```python
from build123d import *

# Parameters (mm, degrees)
SKETCH1_R           = 4.75
BOSS_EXTRUDE1_DEPTH = 5
SKETCH2_R           = 2.25
BOSS_EXTRUDE2_DEPTH = 7.5
BOSS_EXTRUDE3_START = 12.5
SKETCH3_R           = 2.25
BOSS_EXTRUDE3_DEPTH = 12.5
SKETCH4_R           = 1.25
CUT_EXTRUDE1_DEPTH  = 5
CUT_EXTRUDE2_START  = -5
SKETCH5_R           = 1.25
CUT_EXTRUDE2_DEPTH  = 5


with BuildPart() as part:
    # Sketch1 → Boss-Extrude1 (new body)
    with BuildSketch(Plane.XY):
        Circle(SKETCH1_R)
    extrude(amount=BOSS_EXTRUDE1_DEPTH)

    # Sketch2 → Boss-Extrude2 (add)
    with BuildSketch(Plane.XY.offset(5)):
        Circle(SKETCH2_R)
    extrude(amount=BOSS_EXTRUDE2_DEPTH)

    # Sketch3 → Boss-Extrude3 (add)
    with BuildSketch(Plane(origin=(0, 0, 0), x_dir=(-1, 0, 0), z_dir=(0, 0, -1)).offset(BOSS_EXTRUDE3_START)):
        with Locations(Location((0, 0, 0), (0, 0, 180))):
            Circle(SKETCH3_R)
    extrude(amount=-BOSS_EXTRUDE3_DEPTH)

    # Sketch4 → Cut-Extrude1 (cut)
    with BuildSketch(Plane.XY.offset(12.5)):
        Circle(SKETCH4_R)
    extrude(amount=-CUT_EXTRUDE1_DEPTH, mode=Mode.SUBTRACT)

    # Sketch5 → Cut-Extrude2 (cut)
    with BuildSketch(Plane(origin=(0, 0, -12.5), x_dir=(-1, 0, 0), z_dir=(0, 0, -1)).offset(CUT_EXTRUDE2_START)):
        with Locations(Location((0, 0, 0), (0, 0, 180))):
            Circle(SKETCH5_R)
    extrude(amount=CUT_EXTRUDE2_DEPTH, mode=Mode.SUBTRACT)


solid = part.part
```
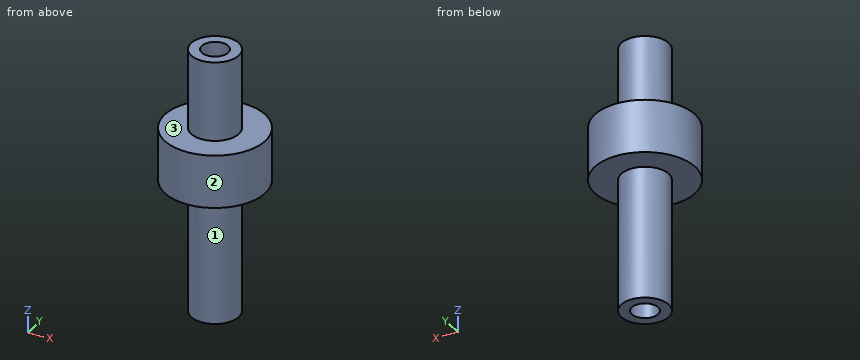
Geometry: final body of the model. Coordinates: model frame, mm. Face numbers are marked on the shaded views. A direction names the side the tool comes from. Round coordinates to 2 decimals unless told otherwise and drop trailing zeros. Write each loop counter-clockwise with the first axis right and the second up, starting at its lowest first coordinate (ties: lowest second). Pieces come first, ordered by that corner, then holes. Notation, with made-up numbers: M 43,10 L 98,10 A10 cw 98,25 Z; hole C 59.5,41.25 d10. An arc over 180 degrees is marked long. Answer in a Markdown table with one row per item. Add a question column.
(1) Cut plane C-C, the plane z = -10.25. Return the cut outline in (x, y), then the cut area to 3 significant figures.
(2) Cut plane A-A, the plane x = 0. Return the cut outline in (y, z).
(3) Cut plane D-D, the plane z = 3.25. Return the cut outline in (x, y).
(4) Ray query, L1, parallel to Y at x = 0, z = -9.6; L2, parallel to Z at x = -3.5, y = -0.75; L3, parallel to X at y = -1.75, z = 7. Return the intervals inside material, ascending.
(5) Contact query for flat-ended pins moving along their axis: pin 1 (1.5 mm diameter, centred on x = 2, z = -2, fed in from +Y); pin 2 (1.5 mm diameter, centred on x = 0, y = 0, fed in from +Z). Output: stop coordinate, or through.
(6) Cut plane B-B, the plane y = 1.5. Return the cut outline in (x, z).
(7) Reachability of the marked faces 1, 2 and 3 from +Z, -Z, +X, -X, +Y, -Y: full face, straight path, thin tool, end or side. Return the list, or none.
Established:
| question | item | result |
|---|---|---|
| 1 | outline | C 0,0 d4.5; hole C 0,0 d2.5 |
| 1 | area | 11.0 mm² |
| 2 | outline | M -4.75,0 L -2.25,0 L -2.25,-12.5 L -1.25,-12.5 L -1.25,-7.5 L 1.25,-7.5 L 1.25,-12.5 L 2.25,-12.5 L 2.25,0 L 4.75,0 L 4.75,5 L 2.25,5 L 2.25,12.5 L 1.25,12.5 L 1.25,7.5 L -1.25,7.5 L -1.25,12.5 L -2.25,12.5 L -2.25,5 L -4.75,5 Z |
| 3 | outline | C 0,0 d9.5 |
| 4 | L1 | -2.25 to -1.25, 1.25 to 2.25 |
| 4 | L2 | 0 to 5 |
| 4 | L3 | -1.41 to 1.41 |
| 5 | pin 1 | y = 1.87 |
| 5 | pin 2 | z = 7.5 |
| 6 | outline | M -4.51,0 L -1.68,0 L -1.68,-12.5 L 1.68,-12.5 L 1.68,0 L 4.51,0 L 4.51,5 L 1.68,5 L 1.68,12.5 L -1.68,12.5 L -1.68,5 L -4.51,5 Z |
| 7 | face 1 | -Z |
| 7 | face 2 | +Z, -Z |
| 7 | face 3 | +Z |
